Work out the finished part from the listing and answer in its coordinate system (mm). A direction names the side the tool comes from. Coordinates: 2 decimals unless noted, no trailing zeros. Order: outer loops, then holes, each group sorted by start corner. A loop starts at its lowest first (then second) coordinate and runs counter-clockwise, first axis right, second up. Notation, with made-up numbers: M 36.5,-7.5 L 75.5,-7.5 A7 cw 75.5,5.5 Z; hole C -12.5,-3 d10. An arc over 180 degrees is marked long. Write item = value, one per line. Start each with the question number.
Q1. Straight lines are drawn through the part: line 1 along Y through (x, z) = (0.5, -2.5); line 2 along Y through (x, z) = (0.75, 0.25); line 3 along Z through (x, y) = (-0.75, 33). For each, find the intervals that lie inside material, in ascending order.
Q2. Find section D-D on z = 3.25. Give the vertices of the cut face in (x, y).
Q3. A tool of negligible diameter and unlimited length cuts with its end or side. For faces 4 (the flat face through (-1, 39, 0)), 5 (the flat face through (2, 37, -1)), from which of +Z, -Z, +X, -X, +Y, -Y can it reach the whole face along a straight path? Write none if from no direction.
Q4. Determine the mould class of faces 1 (the flat face through (1, 39, 0)), 2 (the cylindrical face through (-2, 18, 0)), 3 (the flat face through (0, 0, 0)) for opening direction X: released by +X, released by -X, zero draft, split by the parting line, or undercut.
Q5. Find section B-B on z = 0. Give the vertices of the cut face in (x, y), and give its area (3 significant figures).
Q6. Each of these flat-tipped pins is pushed along its axis until it touches: P1, Ø1, axis at x = 0, z = 1, coming from the +Y side; P2, Ø3, axis at x = -2, y = 29.5, coming from the -Z side; P3, Ø2, axis at y = 39.5, z = -1, coming from the -X side. Where does it stop, or does it pass through?
Q7. Find section A-A on x = 0. Give the vertices of the cut face in (y, z).
Q8. Find section C-C on y = 22. Give the vertices of the cut face in (x, z).
```python
from build123d import *

# Parameters (mm, degrees)
SKETCH1_R               = 2
BOSS_EXTRUDE1_DEPTH     = 37
CUT_EXTRUDE1_DEPTH      = 42.388404173
CUT_EXTRUDE1_DEPTH_BACK = 42.388404173
SKETCH3_W               = 2
SKETCH3_H               = 3.126637596


with BuildPart() as part:
    # Sketch1 → Boss-Extrude1 (new body)
    with BuildSketch(Plane(origin=(0, 0, 0), x_dir=(1, 0, 0), z_dir=(0, 1, 0))):
        with Locations(Location((0, 0, 0), (0, 0, 270))):
            Circle(SKETCH1_R)
    extrude(amount=BOSS_EXTRUDE1_DEPTH)

    # Sketch2 → Revolve1 (revolve)
    with BuildSketch(Plane.XY):
        with BuildLine():
            Line((0, 41), (0, 37))
            Line((0, 37), (4, 37))
            ThreePointArc((4, 37), (2.828427125, 39.828427125), (0, 41))
        make_face()
    revolve(axis=Axis((0, 37, 0), (0, -1, 0)))

    # Sketch3 → Cut-Extrude1 (cut, two sides: drawn at the far end of the back side and taken through both)
    with BuildSketch(Plane.XY.offset(-CUT_EXTRUDE1_DEPTH_BACK)):
        with Locations((0, 39.743318798)):
            Rectangle(SKETCH3_W, SKETCH3_H)
    extrude(amount=CUT_EXTRUDE1_DEPTH + CUT_EXTRUDE1_DEPTH_BACK, mode=Mode.SUBTRACT)


solid = part.part
```
Findings below:
q1.line_1 = 37 to 38.18
q1.line_2 = 0 to 38.18
q1.line_3 = -1.85 to 1.85
q2.outline = M -2.33,37 L 2.33,37 A2.33 ccw 1,39.11 L 1,38.18 L -1,38.18 L -1,39.11 A2.33 ccw Z
q3.face_4 = +Z, -Z, +Y
q3.face_5 = -Y
q4.face_1 = undercut
q4.face_2 = split by the parting line
q4.face_3 = zero draft
q5.outline = M -4,37 L -2,37 L -2,0 L 2,0 L 2,37 L 4,37 A4 ccw 1,40.87 L 1,38.18 L -1,38.18 L -1,40.87 A4 ccw Z
q5.area = 168 mm^2
q6.P1 = 38.18
q6.P2 = -1.94
q6.P3 = -3.62
q7.outline = M 0,-2 L 37,-2 L 37,-4 A4 ccw 38.18,-3.82 L 38.18,3.82 A4 ccw 37,4 L 37,2 L 0,2 Z
q8.outline = C 0,0 d4
